Part model, mm, in its own coordinate system. A direction names the side the tool comes from. Coordinates: 2 decimals unless noted, no trailing zeros. Loops run counter-clockwise (first coordinate to the right, second up) from the corner with the lowest first, then second, coordinate; pieces in that order, holes last. Notation, with made-up numbers: (69, 67) - (116, 67) arc R16 ccw to (116, 77) - close; hole circle Ø9 at (11.25, 47.5). An arc over 180 degrees is marked (long way). Use a Markdown table: item, result. Add a question column.
1) Band-saw the part on A-A (y = 77). Give the cut face in (x, z), plus the area to 3 significant figures.
2) Probe probe 1 along X at (y, z) = (85.25, 42); probe 2 along Y at (x, z) = (-82.9, 23.2); probe 3 along Z at (x, y) = (-61.5, 79.5). List the from-to ranges inside material, lowest first. Write a range as [from, to].
3) Drop flat-ended pins along their axis: P1, Ø12, axis at x = -75, z = 36.5, coming from the -Y side; P2, Ø1.5, axis at x = -78.57, y = 82.95, coming from the -Z side; P3, Ø2, axis at x = -78.57, y = 82.95, coming from the +Z side. Give the stop position or say it passes through.
4) Tool access for faces 1 (the face through (-78.065, 77, 47)), 2 (the face through (-12.065, 77, 15)), 3 (the face through (-0.285, 83.816, 23.751)), 4 (the face through (-78.667, 76.938, 43.77)): list every direction of +Z, -Z, +X, -X, +Y, -Y with a clear straight run to the whole face (end or side of a thin tool).
5) Band-saw the part on B-B (z = 30.2). Give the cut face in (x, y), plus the area to 4 significant figures.
6) Pull direction Y, two halves, no side cores. Call faces 5 (the face through (-17, 80.952, 22)), 6 (the face through (-77.893, 84.006, 15.002)), 7 (the face through (-83.495, 82.008, 11.801)): +Y half, -Y half, draft (parallel to the pull), parting line (faces both ways), or undercut.
7) Band-saw the part on C-C (x = -45). Give the cut face in (y, z), plus the area to 3 significant figures.
8) Band-saw the part on D-D (x = -27.5). Give the cut face in (y, z).
from build123d import *

# Parameters (mm, degrees)
BOSS_EXTRUDE1_DEPTH          = 38
FILLET3_R                    = 2
CUT_EXTRUDE1_DEPTH           = 98.532671663
CUT_EXTRUDE1_DEPTH_BACK      = 98.532671663
M3X0_5_TAPPED_HOLE2_D        = 2.5
M3X0_5_TAPPED_HOLE2_DEPTH    = 7.5
M3X0_5_TAPPED_HOLE2_TIP      = 0.751075774
M3X0_5_TAPPED_HOLE3_D        = 2.5
M3X0_5_TAPPED_HOLE3_DEPTH    = 7.5
M3X0_5_TAPPED_HOLE3_TIP      = 0.751075774
M2_5X0_45_TAPPED_HOLE1_D     = 2.05
M2_5X0_45_TAPPED_HOLE1_DEPTH = 6.35
M2_5X0_45_TAPPED_HOLE1_TIP   = 0.615882135
M2_5X0_45_TAPPED_HOLE2_D     = 2.05
M2_5X0_45_TAPPED_HOLE2_DEPTH = 6.35
M2_5X0_45_TAPPED_HOLE2_TIP   = 0.615882135
SKETCH13_W                   = 6
SKETCH13_H                   = 6
BOSS_EXTRUDE3_DEPTH          = 2
FILLET6_R                    = 2
M3X0_5_TAPPED_HOLE4_D        = 2.5
M3X0_5_TAPPED_HOLE4_DEPTH    = 5.2
M3X0_5_TAPPED_HOLE4_TIP      = 0.751075774


with BuildPart() as part:
    # Sketch2 → Boss-Extrude1 (new body)
    with BuildSketch(Plane.XY.offset(11.2)):
        Polygon((-84.06534388, 85.95185693), (-75.56534388, 85.95185693), (-75.56534388, 80.95185693), (-5.56534388, 80.95185693), (-5.56534388, 85.95185693), (2.93465612, 85.95185693), (2.93465612, 77.95185693), (-84.06534388, 77.95185693), align=None)
    extrude(amount=BOSS_EXTRUDE1_DEPTH)

    # Fillet3
    fillet3_edges = [part.edges().sort_by_distance(p)[0] for p in [
        (2.93465612, 81.95185693, 49.2),
        (-84.06534388, 81.95185693, 11.2),
        (-84.06534388, 81.95185693, 49.2),
        (2.93465612, 81.95185693, 11.2),
    ]]
    fillet(fillet3_edges, radius=FILLET3_R)

    # Sketch3 → Cut-Extrude1 (cut, two sides: drawn at the far end of the back side and taken through both)
    with BuildSketch(Plane(origin=(0, 80.95185693, 0), x_dir=(1, 0, 0), z_dir=(0, 1, 0)).offset(-CUT_EXTRUDE1_DEPTH_BACK)):
        with BuildLine():
            Line((-66.06534388, -15.2), (-30.06534388, -15.2))
            ThreePointArc((-30.06534388, -15.2), (-15.06534388, -30.2), (-30.06534388, -45.2))
            Line((-30.06534388, -45.2), (-66.06534388, -45.2))
            ThreePointArc((-66.06534388, -45.2), (-81.06534388, -30.2), (-66.06534388, -15.2))
        make_face()
    extrude(amount=CUT_EXTRUDE1_DEPTH + CUT_EXTRUDE1_DEPTH_BACK, mode=Mode.SUBTRACT)

    # M3x0.5 Tapped Hole2
    with Locations(Plane(origin=(0, 0, 11.2), x_dir=(-1, 0, 0), z_dir=(0, 0, -1))):
        with Locations((78.56534388, 82.95185693), (2.56534388, 82.95185693)):
            Hole(M3X0_5_TAPPED_HOLE2_D / 2, depth=M3X0_5_TAPPED_HOLE2_DEPTH)
            with Locations((0, 0, -(M3X0_5_TAPPED_HOLE2_DEPTH + M3X0_5_TAPPED_HOLE2_TIP / 2))):  # 118° drill point
                Cone(0, M3X0_5_TAPPED_HOLE2_D / 2, M3X0_5_TAPPED_HOLE2_TIP, mode=Mode.SUBTRACT)

    # M3x0.5 Tapped Hole3
    with Locations(Plane.XY.offset(49.2)):
        with Locations((-2.56534388, 82.95185693), (-78.56534388, 82.95185693)):
            Hole(M3X0_5_TAPPED_HOLE3_D / 2, depth=M3X0_5_TAPPED_HOLE3_DEPTH)
            with Locations((0, 0, -(M3X0_5_TAPPED_HOLE3_DEPTH + M3X0_5_TAPPED_HOLE3_TIP / 2))):  # 118° drill point
                Cone(0, M3X0_5_TAPPED_HOLE3_D / 2, M3X0_5_TAPPED_HOLE3_TIP, mode=Mode.SUBTRACT)

    # M2.5x0.45 Tapped Hole1
    with Locations(Plane.ZY.offset(84.06534388)):
        with Locations((37.2, 82.95185693), (23.2, 82.95185693)):
            Hole(M2_5X0_45_TAPPED_HOLE1_D / 2, depth=M2_5X0_45_TAPPED_HOLE1_DEPTH)
            with Locations((0, 0, -(M2_5X0_45_TAPPED_HOLE1_DEPTH + M2_5X0_45_TAPPED_HOLE1_TIP / 2))):  # 118° drill point
                Cone(0, M2_5X0_45_TAPPED_HOLE1_D / 2, M2_5X0_45_TAPPED_HOLE1_TIP, mode=Mode.SUBTRACT)

    # M2.5x0.45 Tapped Hole2
    with Locations(Plane(origin=(2.93465612, 0, 0), x_dir=(0, 0, -1), z_dir=(1, 0, 0))):
        with Locations((-23.2, 82.95185693), (-37.2, 82.95185693)):
            Hole(M2_5X0_45_TAPPED_HOLE2_D / 2, depth=M2_5X0_45_TAPPED_HOLE2_DEPTH)
            with Locations((0, 0, -(M2_5X0_45_TAPPED_HOLE2_DEPTH + M2_5X0_45_TAPPED_HOLE2_TIP / 2))):  # 118° drill point
                Cone(0, M2_5X0_45_TAPPED_HOLE2_D / 2, M2_5X0_45_TAPPED_HOLE2_TIP, mode=Mode.SUBTRACT)

    # Sketch13 → Boss-Extrude3 (add)
    with BuildSketch(Plane.XZ.offset(-77.95185693)):
        with Locations((-81.06534388, 14.2)):
            Rectangle(SKETCH13_W, SKETCH13_H)
        with Locations((-81.06534388, 46.2)):
            Rectangle(SKETCH13_W, SKETCH13_H)
        with Locations((-15.06534388, 14.2)):
            Rectangle(SKETCH13_W, SKETCH13_H)
        with Locations((-15.06534388, 46.2)):
            Rectangle(SKETCH13_W, SKETCH13_H)
    extrude(amount=BOSS_EXTRUDE3_DEPTH)

    # Fillet6
    fillet6_edges = [part.edges().sort_by_distance(p)[0] for p in [
        (-12.06534388, 76.95185693, 49.2),
        (-12.06534388, 76.95185693, 11.2),
        (-84.06534388, 76.95185693, 11.2),
        (-84.06534388, 76.95185693, 49.2),
        (-78.06534388, 76.95185693, 17.2),
        (-78.06534388, 76.95185693, 43.2),
        (-18.06534388, 76.95185693, 43.2),
        (-18.06534388, 76.95185693, 17.2),
    ]]
    fillet(fillet6_edges, radius=FILLET6_R)

    # M3x0.5 Tapped Hole4
    with Locations(Plane.XZ.offset(-75.95185693)):
        with Locations((-15.06534388, 46.2), (-15.06534388, 14.2), (-81.06534388, 14.2), (-81.06534388, 46.2)):
            Hole(M3X0_5_TAPPED_HOLE4_D / 2, depth=M3X0_5_TAPPED_HOLE4_DEPTH)
            with Locations((0, 0, -(M3X0_5_TAPPED_HOLE4_DEPTH + M3X0_5_TAPPED_HOLE4_TIP / 2))):  # 118° drill point
                Cone(0, M3X0_5_TAPPED_HOLE4_D / 2, M3X0_5_TAPPED_HOLE4_TIP, mode=Mode.SUBTRACT)


solid = part.part
Answer block:
| question | item | result |
|---|---|---|
| 1 | outline | (-84.07, 13.2) arc R2 ccw to (-82.07, 11.2) - (-78.07, 11.2) - (-78.07, 15.2) arc R2 ccw to (-80.07, 17.2) - (-84.07, 17.2) - close; (-84.07, 43.2) - (-80.07, 43.2) arc R2 ccw to (-78.07, 45.2) - (-78.07, 49.2) - (-82.07, 49.2) arc R2 ccw to (-84.07, 47.2) - close; (-18.07, 11.2) - (-14.07, 11.2) arc R2 ccw to (-12.07, 13.2) - (-12.07, 17.2) - (-16.07, 17.2) arc R2 ccw to (-18.07, 15.2) - close; (-18.07, 45.2) arc R2 ccw to (-16.07, 43.2) - (-12.07, 43.2) - (-12.07, 47.2) arc R2 ccw to (-14.07, 49.2) - (-18.07, 49.2) - close; hole circle Ø2.5 at (-81.07, 14.2); hole circle Ø2.5 at (-81.07, 46.2); hole circle Ø2.5 at (-15.07, 14.2); hole circle Ø2.5 at (-15.07, 46.2) |
| 1 | area | 117 mm2 |
| 2 | probe 1 | [-84.07, -75.57], [-5.57, 2.93] |
| 2 | probe 2 | [77.95, 81.93], [83.98, 85.95] |
| 2 | probe 3 | [11.2, 15.2], [45.2, 49.2] |
| 3 | P1 | y = 77.95 |
| 3 | P2 | z = 19 |
| 3 | P3 | z = 41.55 |
| 4 | face 1 | +Z, -Z, -Y |
| 4 | face 2 | +Z, -Z, +X, -Y |
| 4 | face 3 | +X |
| 4 | face 4 | -Y |
| 5 | outline | (-84.07, 77.95) - (-81.07, 77.95) - (-81.07, 85.95) - (-84.07, 85.95) - close; (-15.07, 77.95) - (2.93, 77.95) - (2.93, 85.95) - (-5.57, 85.95) - (-5.57, 80.95) - (-15.07, 80.95) - close |
| 5 | area | 120.5 mm2 |
| 6 | face 5 | +Y half |
| 6 | face 6 | undercut |
| 6 | face 7 | draft |
| 7 | outline | (77.95, 11.2) - (80.95, 11.2) - (80.95, 15.2) - (77.95, 15.2) - close; (77.95, 45.2) - (80.95, 45.2) - (80.95, 49.2) - (77.95, 49.2) - close |
| 7 | area | 24.0 mm2 |
| 8 | outline | (77.95, 11.2) - (80.95, 11.2) - (80.95, 15.42) - (77.95, 15.42) - close; (77.95, 44.98) - (80.95, 44.98) - (80.95, 49.2) - (77.95, 49.2) - close |
